Read the model definition and answer for the solid it produces. Units are mm, in the model's axes. A direction names the side the tool comes from. Coordinates: 2 decimals unless noted, no trailing zeros. Write each loop counter-clockwise with the first axis right and the second up, starting at its lowest first coordinate (ties: lowest second). Pieces come first, ordered by that corner, then holes. Notation, with made-up numbers: (74, 18) -> (82, 18) arc R30 cw to (82, 53) -> close; hole circle Ø10 at (83, -14.5). An arc over 180 degrees is marked (long way). Return JSON: item names as keys, results as strings.
Autodesk Inventor part; units mm, degrees
ref_plane "Arbeitsebene1" through (90, 0, 250) normal (1, 0, 0) x (0, 0, -1)
ref_plane "YZ Plane" through (0, 0, 0) normal (1, 0, 0) x (0, 1, 0)
ref_plane "XZ Plane" through (0, 0, 0) normal (0, 1, 0) x (-1, 0, 0)
sketch "Skizze1" plane through (0, 0, 0) normal (0, 1, 0) x (-1, 0, 0)
  point P0 (0, 0)
sketch "Skizze2" plane through (0, 0, 0) normal (0, 1, 0) x (-1, 0, 0)
  line L0 (0, 0) -> (-180, 0)
  line L1 (-180, 0) -> (-180, 250)
  line L2 (-180, 250) -> (0, 250)
  line L3 (0, 250) -> (0, 0)
  dimension "d0" = 180
  dimension "d1" = 250
extrude "Extrusion1" add sketch "Skizze2" along normal blind 15
sketch "Skizze3" plane through (0, 15, 0) normal (0, 1, 0) x (1, 0, 0)
  line L0 (10.7918, -15) -> (38.4358, -15)
  line L1 (38.4358, -15) -> (38.4358, -235)
  line L2 (38.4358, -235) -> (10.7918, -235)
  line L3 (10.7918, -235) -> (10.7918, -15)
  line L4 (0, -250) -> (180, -250)
  point P0 (0, 0)
  point P1 (24.6138, -15)
  point P2 (24.6138, -235)
  dimension "d79" = 220
  dimension "d80" = 15
extrude "Extrusion2" cut sketch "Skizze3" against normal blind 10
sketch "Skizze4" plane through (0, 15, 0) normal (0, 1, 0) x (1, 0, 0)
  line L0 (54.0028, -52.3007) -> (130.0028, -52.3007)
  line L1 (130.0028, -52.3007) -> (130.0028, -96.3007)
  line L2 (130.0028, -96.3007) -> (54.0028, -96.3007)
  line L3 (54.0028, -96.3007) -> (54.0028, -52.3007)
  point P0 (0, 0)
  dimension "d6" = 76
  dimension "d7" = 44
extrude "Extrusion3" add sketch "Skizze4" along normal blind 5
sketch "Skizze5" plane through (0, 15, 0) normal (0, 1, 0) x (1, 0, 0)
  line L0 (56.8154, -93.8586) -> (61.8154, -93.8586)
  line L1 (61.8154, -93.8586) -> (61.8154, -88.8586)
  line L2 (61.8154, -88.8586) -> (56.8154, -88.8586)
  line L3 (56.8154, -88.8586) -> (56.8154, -93.8586)
  line L4 (56.8154, -55.8667) -> (61.8154, -55.8667)
  line L5 (61.8154, -55.8667) -> (61.8154, -60.8667)
  line L6 (61.8154, -60.8667) -> (56.8154, -60.8667)
  line L7 (56.8154, -60.8667) -> (56.8154, -55.8667)
  point P0 (0, 0)
  dimension "d10" = 5
  dimension "d11" = 5
  dimension "d12" = 5
extrude "Extrusion4" add sketch "Skizze5" along normal blind 6 contours L3 L2 L1 L0
sketch "Skizze6" plane through (0, 20, 0) normal (0, 1, 0) x (1, 0, 0)
  line L0 (61.8154, -59.6582) -> (56.8154, -59.6582)
  line L1 (56.8154, -59.6582) -> (56.8154, -54.6582)
  line L2 (56.8154, -54.6582) -> (61.8154, -54.6582)
  line L3 (61.8154, -54.6582) -> (61.8154, -59.6582)
  point P0 (0, 0)
  dimension "d15" = 5
extrude "Extrusion5" add sketch "Skizze6" along normal blind 1
sketch "Skizze7" plane through (0, 20, 0) normal (0, 1, 0) x (1, 0, 0)
  line L0 (121.8231, -54.6582) -> (126.8231, -54.6582)
  line L1 (126.8231, -54.6582) -> (126.8231, -59.6582)
  line L2 (126.8231, -59.6582) -> (121.8231, -59.6582)
  line L3 (121.8231, -59.6582) -> (121.8231, -54.6582)
  point P0 (0, 0)
  dimension "d18" = 5
extrude "Extrusion6" add sketch "Skizze7" along normal blind 1
sketch "Skizze8" plane through (0, 20, 0) normal (0, 1, 0) x (1, 0, 0)
  line L0 (122.1095, -93.6637) -> (127.1095, -93.6637)
  line L1 (127.1095, -93.6637) -> (127.1095, -88.6637)
  line L2 (127.1095, -88.6637) -> (122.1095, -88.6637)
  line L3 (122.1095, -88.6637) -> (122.1095, -93.6637)
  point P0 (0, 0)
  point P1 (124.6095, -93.6637)
  point P2 (124.6095, -88.6637)
  dimension "d21" = 5
  dimension "d22" = 5
extrude "Extrusion7" add sketch "Skizze8" along normal blind 1
sketch "Skizze9" plane through (0, 15, 0) normal (0, 1, 0) x (1, 0, 0)
  line L0 (54.0028, -106.6154) -> (124.8609, -106.6154)
  line L1 (124.8609, -106.6154) -> (124.8609, -136.072)
  line L2 (124.8609, -136.072) -> (54.0028, -136.072)
  line L3 (54.0028, -136.072) -> (54.0028, -106.6154)
  line L4 (130.0028, -52.3007) -> (54.0028, -52.3007)
  line L5 (54.0028, -96.3007) -> (130.0028, -96.3007)
  line L6 (0, -250) -> (180, -250)
  point P0 (0, 0)
  point P1 (89.4318, -136.072)
  dimension "d182" = 83.7713
  dimension "d183" = 10.3146
  dimension "d184" = 113.928
  dimension "d185" = 113.928
extrude "Extrusion8" add sketch "Skizze9" along normal blind 5
sketch "Skizze10" plane through (0, 20, 0) normal (0, 1, 0) x (1, 0, 0)
  line L0 (57.3891, -109.317) -> (59.9809, -109.317)
  line L1 (59.9809, -109.317) -> (59.9809, -134.3091)
  line L2 (59.9809, -134.3091) -> (57.3891, -134.3091)
  line L3 (57.3891, -134.3091) -> (57.3891, -109.317)
  point P0 (0, 0)
extrude "Extrusion9" add sketch "Skizze10" along normal blind 1
sketch "Skizze11" plane through (0, 20, 0) normal (0, 1, 0) x (1, 0, 0)
  line L0 (121.6279, -109.6873) -> (119.2213, -109.6873)
  line L1 (119.2213, -109.6873) -> (119.2213, -133.7537)
  line L2 (119.2213, -133.7537) -> (121.6279, -133.7537)
  line L3 (121.6279, -133.7537) -> (121.6279, -109.6873)
  point P0 (0, 0)
extrude "Extrusion10" add sketch "Skizze11" along normal blind 1
sketch "Skizze14" plane through (0, 5, 0) normal (0, 1, 0) x (1, 0, 0)
  line L0 (10.7918, -235) -> (10.7918, -15)
  line L1 (38.4358, -15) -> (38.4358, -235)
  line L2 (10.7918, -15) -> (38.4358, -15)
  line L3 (38.4358, -15) -> (38.4358, -35)
  line L4 (38.4358, -35) -> (10.7918, -35)
  line L5 (10.7918, -35) -> (10.7918, -15)
  line L6 (10.7918, -55) -> (38.4358, -55)
  line L7 (38.4358, -55) -> (38.4358, -75)
  line L8 (38.4358, -75) -> (10.7918, -75)
  line L9 (10.7918, -75) -> (10.7918, -55)
  line L10 (10.7918, -95) -> (38.4358, -95)
  line L11 (38.4358, -95) -> (38.4358, -115)
  line L12 (38.4358, -115) -> (10.7918, -115)
  line L13 (10.7918, -115) -> (10.7918, -95)
  line L14 (10.7918, -135) -> (38.4358, -135)
  line L15 (38.4358, -135) -> (38.4358, -155)
  line L16 (38.4358, -155) -> (10.7918, -155)
  line L17 (10.7918, -155) -> (10.7918, -135)
  line L18 (10.7918, -175) -> (38.4358, -175)
  line L19 (38.4358, -175) -> (38.4358, -195)
  line L20 (38.4358, -195) -> (10.7918, -195)
  line L21 (10.7918, -195) -> (10.7918, -175)
  line L22 (10.7918, -215) -> (38.4358, -215)
  line L23 (38.4358, -215) -> (38.4358, -235)
  line L24 (38.4358, -235) -> (10.7918, -235)
  line L25 (10.7918, -235) -> (10.7918, -215)
  point P0 (0, 0)
  point P1 (24.6138, -55)
  point P2 (24.6138, -35)
  point P3 (24.6138, -95)
  point P4 (24.6138, -135)
  point P5 (24.6138, -175)
  point P6 (24.6138, -155)
  point P7 (24.6138, -215)
  point P8 (24.6138, -195)
  point P9 (10.7918, -235)
  point P10 (38.4358, -215)
  point P11 (10.7918, -195)
  point P12 (38.4358, -175)
  point P13 (10.7918, -155)
  point P14 (38.4358, -135)
  point P15 (10.7918, -115)
  point P16 (38.4358, -95)
  point P17 (10.7918, -75)
  point P18 (38.4358, -55)
  point P19 (10.7918, -55)
  point P20 (10.7918, -35)
  dimension "d42" = 20
  dimension "d43" = 20
  dimension "d44" = 20
  dimension "d45" = 20
  dimension "d46" = 20
  dimension "d47" = 20
  dimension "d48" = 20
  dimension "d49" = 20
  dimension "d50" = 20
  dimension "d51" = 20
  dimension "d52" = 20
extrude "Extrusion12" cut sketch "Skizze14" against normal blind 20 contours L0 L22 L1 L24 | L0 L18 L1 L20 | L0 L14 L1 L16 | L0 L10 L1 L12 | L0 L6 L1 L8 | L0 L2 L1 L4
ref_plane "Arbeitsebene1" through (90, 0, 250) normal (1, 0, 0) x (0, 0, -1)
mirror "Spiegeln1" about plane through (90, 0, 250) normal (1, 0, 0) of "Extrusion12"
mirror "Spiegeln2" about plane through (90, 0, 250) normal (1, 0, 0) of "Extrusion2"
sketch "Skizze15" plane through (0, 15, 0) normal (0, 1, 0) x (1, 0, 0)
  line L0 (55, -210) -> (65, -210)
  line L1 (65, -210) -> (65, -200)
  line L2 (65, -200) -> (55, -200)
  line L3 (55, -200) -> (55, -210)
  line L4 (115, -210) -> (125, -210)
  line L5 (125, -210) -> (125, -200)
  line L6 (125, -200) -> (115, -200)
  line L7 (115, -200) -> (115, -210)
  line L8 (0, -250) -> (180, -250)
  line L9 (55, -50) -> (65, -50)
  line L10 (65, -50) -> (65, -40)
  line L11 (65, -40) -> (55, -40)
  line L12 (55, -40) -> (55, -50)
  line L13 (115, -50) -> (125, -50)
  line L14 (125, -50) -> (125, -40)
  line L15 (125, -40) -> (115, -40)
  line L16 (115, -40) -> (115, -50)
  line L17 (0, 0) -> (0, -250)
  line L18 (180, -250) -> (180, 0)
  line L19 (180, 0) -> (0, 0)
  point P0 (120, -210)
  point P1 (60, -50)
  point P2 (120, -50)
  point P3 (55, -205)
  point P4 (125, -205)
  point P5 (55, -45)
  point P6 (125, -45)
  point P7 (60, -210)
  point P8 (60, -40)
  point P9 (120, -40)
  dimension "d56" = 10
  dimension "d57" = 10
  dimension "d58" = 10
  dimension "d59" = 10
  dimension "d60" = 40
  dimension "d61" = 10
  dimension "d62" = 10
  dimension "d63" = 10
  dimension "d64" = 10
  dimension "d72" = 55
  dimension "d73" = 55
  dimension "d74" = 55
  dimension "d75" = 55
  dimension "d76" = 40
  dimension "d77" = 40
  dimension "d78" = 40
extrude "Extrusion13" cut sketch "Skizze15" against normal blind 20 contours L3 L2 L1 L0 | L7 L6 L5 L4 | L12 L11 L10 L9 | L16 L15 L14 L13
fillet "Rundung9" radius 8 4 edges at (180, 7.5, 250) (180, 7.5, 0) (0, 7.5, 0) (0, 7.5, 250)
properties part number "WRO Modell_RC_Auto_3"
1. A tool of negligible diameter and unlimited length cuts with its end or side. For faces 3 (the face through (59, 21, 57)), 4 (the face through (24, 3, 55)), 5 (the face through (93, 17, 96.301)), 6 (the face through (180, 7, 123)), 7 (the face through (24, 5, 205)), from which of +Z, -Z, +X, -X, +Y, -Y can it reach the whole face along a straight path? Write none if from no direction.
Taken from the geometry:
{"face 3": "+Z, -Z, +X, -X, +Y", "face 4": "+Y, -Y", "face 5": "+X, -X, +Y", "face 6": "+Z, -Z, +X, +Y, -Y", "face 7": "+Y"}
2. Flat-ended cylindrical pins translate along their axes: pin 1 Ø6 at (x, z) = (159.5, 49) entering from +Y; pin 2 Ø0.8 at (y, z) = (20.5, 121) entering from -X; pin 3 Ø0.5 at (x, y) = (125.5, 20.5) entering from +Z. Find the tip coordinate at first contact, or state that the pin passes through.
Taken from the geometry:
{"pin 1": "stops at y = 5", "pin 2": "stops at x = 57.39", "pin 3": "stops at z = 93.66"}
3. For a pull along Z with two mould halves and no side action, classify faces 1 (the face through (120, 8, 210)), 2 (the face through (54.003, 17, 75)) as +Z half, -Z half, draft (parallel to the pull), parting line (faces both ways), or undercut.
Taken from the geometry:
{"face 1": "undercut", "face 2": "draft"}
4. The part is cut by section C-C (y = 12). Count the separate pieces of the cut face and the enclosed holes in it, then the cut area to 3 significant figures.
Taken from the geometry:
{"separate pieces": "1", "enclosed holes": "6", "area": "32,400 mm2"}
5. The part is cut by section A-A (x = 148). Determine the outline of the cut face in (y, z).
Taken from the geometry:
{"outline": "(0, 0) -> (15, 0) -> (15, 15) -> (0, 15) -> close; (0, 35) -> (5, 35) -> (5, 55) -> (0, 55) -> close; (0, 75) -> (5, 75) -> (5, 95) -> (0, 95) -> close; (0, 115) -> (5, 115) -> (5, 135) -> (0, 135) -> close; (0, 155) -> (5, 155) -> (5, 175) -> (0, 175) -> close; (0, 195) -> (5, 195) -> (5, 215) -> (0, 215) -> close; (0, 235) -> (15, 235) -> (15, 250) -> (0, 250) -> close"}
6. The part is cut by section B-B (z = 145.5). Determine the outline of the cut face in (x, y).
Taken from the geometry:
{"outline": "(0, 0) -> (10.79, 0) -> (10.79, 15) -> (0, 15) -> close; (38.44, 0) -> (141.56, 0) -> (141.56, 15) -> (38.44, 15) -> close; (169.21, 0) -> (180, 0) -> (180, 15) -> (169.21, 15) -> close"}
7. Consider L1, parallel to X at y = 12, z = 136.5; L2, parallel to X at y = 10.75, z = 46.5; L3, parallel to Z at x = 119, y = 4.5. Determine where each line is inside the solid, lowest interval first.
Taken from the geometry:
{"L1": "x = 0 to 10.79, 38.44 to 141.56, 169.21 to 180", "L2": "x = 0 to 10.79, 38.44 to 55, 65 to 115, 125 to 141.56, 169.21 to 180", "L3": "z = 0 to 40, 50 to 200, 210 to 250"}
8. The part is cut by section D-D (x = 91). Determine the outline of the cut face in (y, z), then the cut area to 3 significant figures.
Taken from the geometry:
{"outline": "(0, 0) -> (15, 0) -> (15, 52.3) -> (20, 52.3) -> (20, 96.3) -> (15, 96.3) -> (15, 106.62) -> (20, 106.62) -> (20, 136.07) -> (15, 136.07) -> (15, 250) -> (0, 250) -> close", "area": "4,120 mm2"}
